Part model, mm, in its own coordinate system. Face numbers are marked on the shaded views. Give positions to 0.01 mm unless a question says otherwise; leave off trailing zeros. Write each loop counter-clockwise with the first axis right and the second up, starting at its lowest first coordinate (ties: lowest second). Pieces come first, ordered by that corner, then holes. Notation, with made-up numbers: M 3,-31 L 34,-31 A20 ccw 34,-24 Z; hole C -4.75,69.5 d10. An arc over 180 degrees is marked long. Use a Markdown table: item, result. Add a question column.
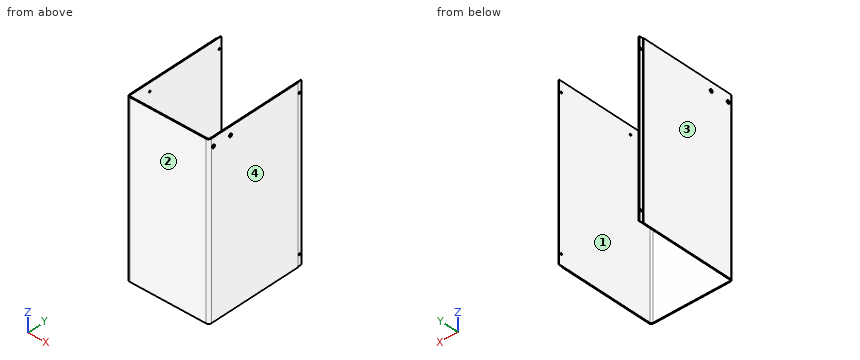
from build123d import *

# Parameters (mm, degrees)
SKETCH1_W                                      = 150
SKETCH1_H                                      = 318.3528
BASE_FLANGE1_DEPTH                             = 2.032
EDGE_FLANGE1_STRIP_W                           = 14.224
EDGE_FLANGE1_STRIP_H                           = 2.032
EDGE_FLANGE1_STRIP_CUT_DEPTH                   = 318.3528
EDGE_FLANGE1_STRIP_2_W                         = 14.224
EDGE_FLANGE1_STRIP_2_H                         = 2.032
EDGE_FLANGE1_STRIP_CUT_2_DEPTH                 = 318.3528
EDGE_FLANGE1_DEPTH                             = 318.3528
EDGE_FLANGE1_BEND_DEPTH                        = 318.3528
SKETCH9_W                                      = 318.3528
SKETCH9_H                                      = 8
CUT_EXTRUDE1_DEPTH                             = 1.016
SKETCH10_W                                     = 318.3528
SKETCH10_H                                     = 8
CUT_EXTRUDE3_DEPTH                             = 1.016
M3_CLEARANCE_HOLE1_D                           = 3.4
CSK_FOR_M3_FLAT_HEAD_MACHINE_SCREW1_AT_2_COUNT = 2
CSK_FOR_M3_FLAT_HEAD_MACHINE_SCREW1_AT_2_PITCH = 35
CSK_FOR_M3_FLAT_HEAD_MACHINE_SCREW2_AT_2_COUNT = 2
CSK_FOR_M3_FLAT_HEAD_MACHINE_SCREW2_AT_2_PITCH = 35


# Sheet-metal steps are written as plain solids
with BuildPart() as part:
    # Sketch1 → Base-Flange1 (new body)
    with BuildSketch(Plane(origin=(0, 0, 0), x_dir=(1, 0, 0), z_dir=(0, 1, 0))):
        with Locations((75, 159.1764)):
            Rectangle(SKETCH1_W, SKETCH1_H)
    extrude(amount=-BASE_FLANGE1_DEPTH)

    # Edge-Flange1 strip (across the edge) → Edge-Flange1 strip cut (cut)
    with BuildSketch(Plane(origin=(150, 0, 0), x_dir=(-1, 0, 0), z_dir=(0, 0, -1))):
        with Locations((-4.064, -1.016)):
            Rectangle(EDGE_FLANGE1_STRIP_W, EDGE_FLANGE1_STRIP_H)
    extrude(amount=EDGE_FLANGE1_STRIP_CUT_DEPTH, mode=Mode.SUBTRACT)

    # Edge-Flange1 strip 2 (across the edge) → Edge-Flange1 strip cut 2 (cut)
    with BuildSketch(Plane.XY.offset(-318.3528)):
        with Locations((-4.064, -1.016)):
            Rectangle(EDGE_FLANGE1_STRIP_2_W, EDGE_FLANGE1_STRIP_2_H)
    extrude(amount=EDGE_FLANGE1_STRIP_CUT_2_DEPTH, mode=Mode.SUBTRACT)

    # Edge-Flange1 section (across the edge) → Edge-Flange1 (add)
    with BuildSketch(Plane(origin=(150, 0, 0), x_dir=(-1, 0, 0), z_dir=(0, 0, -1))):
        with BuildLine():
            Line((-2.032, 3.048), (-2.032, 189.048))
            Line((-2.032, 189.048), (0, 189.048))
            Line((0, 189.048), (0, 3.048))
            ThreePointArc((0, 3.048), (0.892738531, 0.892738531), (3.048, 0))
            Line((3.048, 0), (3.048, -2.032))
            ThreePointArc((3.048, -2.032), (-0.544102448, -0.544102448), (-2.032, 3.048))
        make_face()
    extrude(amount=EDGE_FLANGE1_DEPTH)

    # Edge-Flange1 section 2 (across the edge) → Edge-Flange1 bend (add)
    with BuildSketch(Plane.XY.offset(-318.3528)):
        with BuildLine():
            Line((-2.032, 3.048), (-2.032, 189.048))
            Line((-2.032, 189.048), (0, 189.048))
            Line((0, 189.048), (0, 3.048))
            ThreePointArc((0, 3.048), (0.892738531, 0.892738531), (3.048, 0))
            Line((3.048, 0), (3.048, -2.032))
            ThreePointArc((3.048, -2.032), (-0.544102448, -0.544102448), (-2.032, 3.048))
        make_face()
    extrude(amount=EDGE_FLANGE1_BEND_DEPTH)

    # Sketch9 → Cut-Extrude1 (cut)
    with BuildSketch(Plane(origin=(152.032, 0, 0), x_dir=(0, 0, -1), z_dir=(1, 0, 0))):
        with Locations((159.1764, 185.048)):
            Rectangle(SKETCH9_W, SKETCH9_H)
    extrude(amount=-CUT_EXTRUDE1_DEPTH, mode=Mode.SUBTRACT)

    # Sketch10 → Cut-Extrude3 (cut)
    with BuildSketch(Plane(origin=(-2.032, 0, -3.175), x_dir=(0, 0, -1), z_dir=(1, 0, 0))):
        with Locations((156.0014, 185.048)):
            Rectangle(SKETCH10_W, SKETCH10_H)
    extrude(amount=CUT_EXTRUDE3_DEPTH, mode=Mode.SUBTRACT)

    # M3 Clearance Hole1 (through all)
    with Locations(Plane(origin=(151.016, 0, 0), x_dir=(0, 0, -1), z_dir=(1, 0, 0))):
        with Locations((20.003324657, 185.048), (298.3528, 185.048)):
            Hole(M3_CLEARANCE_HOLE1_D / 2)

    # Sketch20 → CSK for M3 Flat Head Machine Screw1 (revolve, cut)
    with BuildSketch(Plane(origin=(152.032, 42.5, -15.7004), x_dir=(0, 0, -1), z_dir=(0, 1, 0))):
        Polygon((0, 0), (0, 2.032), (1.7, 2.032), (1.7, 1.45), (3.15, 0), align=None)
    csk_for_m3_flat_head_machine_screw1 = revolve(axis=Axis((158.382, 42.5, -15.7004), (-1, 0, 0)), mode=Mode.SUBTRACT)

    # CSK for M3 Flat Head Machine Screw1 at 2: CSK for M3 Flat Head Machine Screw1 ×2
    with Locations(*[(0, -i * CSK_FOR_M3_FLAT_HEAD_MACHINE_SCREW1_AT_2_PITCH, 0) for i in range(1, CSK_FOR_M3_FLAT_HEAD_MACHINE_SCREW1_AT_2_COUNT)]):
        add(csk_for_m3_flat_head_machine_screw1, mode=Mode.SUBTRACT)

    # Sketch23 → CSK for M3 Flat Head Machine Screw2 (revolve, cut)
    with BuildSketch(Plane(origin=(-2.032, 42.5, -15.7004), x_dir=(0, 0, 1), z_dir=(0, 1, 0))):
        Polygon((0, 0), (0, 2.032), (1.7, 2.032), (1.7, 1.45), (3.15, 0), align=None)
    csk_for_m3_flat_head_machine_screw2 = revolve(axis=Axis((-8.382, 42.5, -15.7004), (1, 0, 0)), mode=Mode.SUBTRACT)

    # CSK for M3 Flat Head Machine Screw2 at 2: CSK for M3 Flat Head Machine Screw2 ×2
    with Locations(*[(0, -i * CSK_FOR_M3_FLAT_HEAD_MACHINE_SCREW2_AT_2_PITCH, 0) for i in range(1, CSK_FOR_M3_FLAT_HEAD_MACHINE_SCREW2_AT_2_COUNT)]):
        add(csk_for_m3_flat_head_machine_screw2, mode=Mode.SUBTRACT)


solid = part.part
1. Mould opens along X. For the marked faces 1, 2, 3 and 4 say: released by +X, released by -X, zero draft, split by the parting line, or undercut.
2. Cut at C-C (x = 39.5). Write the cut outline in (y, z).
3. Cut at B-B (z = -249). Write the cut outline in (x, y), then the cut area to 3 significant figures.
4. Drill centre lines: probe 1 along X at (y, z) = (57, -199); probe 2 along Y at (x, z) = (39.5, -107). Where is each one in solid material? Low to high. Write a range as [from, to].
5. Flat gauge pins, fed straight in: pin 1 (2 mm diameter, centred on y = 42.5, z = -15.7, fed in from +X); pin 2 (3 mm diameter, centred on x = 38, z = -250.5, fed in from +Y); pin 3 (9 mm diameter, centred on y = 186.5, z = -172.5, fed in from -X); pin 4 (5.5 mm diameter, centred on y = 185.05, z = -20, fed in from +X). Where does each tip first touch, or does it go through?
6. Cut at A-A (y = 111.5). Write the cut outline in (x, z), then the cut area to 3 significant figures.
A:
| question | item | result |
|---|---|---|
| 1 | face 1 | undercut |
| 1 | face 2 | zero draft |
| 1 | face 3 | released by -X |
| 1 | face 4 | released by +X |
| 2 | outline | M -2.03,-318.35 L 0,-318.35 L 0,0 L -2.03,0 Z |
| 3 | outline | M -2.03,3.05 A5.08 ccw 3.05,-2.03 L 146.95,-2.03 A5.08 ccw 152.03,3.05 L 152.03,181.05 L 151.02,181.05 L 151.02,189.05 L 150,189.05 L 150,3.05 A3.05 cw 146.95,0 L 3.05,0 A3.05 cw 0,3.05 L 0,189.05 L -1.02,189.05 L -1.02,181.05 L -2.03,181.05 Z |
| 3 | area | 1,060 mm² |
| 4 | probe 1 | x = [-2.03, 0], [150, 152.03] |
| 4 | probe 2 | y = [-2.03, 0] |
| 5 | pin 1 | passes through |
| 5 | pin 2 | stops at y = 0 |
| 5 | pin 3 | stops at x = -1.02 |
| 5 | pin 4 | stops at x = 151.02 |
| 6 | outline | M -2.03,-318.35 L 0,-318.35 L 0,0 L -2.03,0 Z; M 150,-318.35 L 152.03,-318.35 L 152.03,0 L 150,0 Z |
| 6 | area | 1,290 mm² |
